from build123d import *

# Parameters (mm, degrees)
F0_W     = 82.55
F0_H     = 69.85
F1_DEPTH = 2.032
F2_W     = 1.524
F2_H     = 69.85
F3_DEPTH = 1.016
F5_DEPTH = 88.8746


with BuildPart() as f1:
    # F0 (on Top) → F1 (new body)
    with BuildSketch(Plane.XY):
        with Locations((-16.0199867169, 0.6959252059)):
            Rectangle(F0_W, F0_H)
    extrude(amount=F1_DEPTH)

    # F2 (on face) → F3 (join)
    with BuildSketch(Plane.XY.offset(2.032)):
        with Locations((-56.5329867169, 0.6959252059)):
            Rectangle(F2_W, F2_H)
        with Locations((-47.5413867169, 0.6959252059)):
            Rectangle(F2_W, F2_H)
        with Locations((-38.5497867169, 0.6959252059)):
            Rectangle(F2_W, F2_H)
        with Locations((-29.5581867169, 0.6959252059)):
            Rectangle(F2_W, F2_H)
        with Locations((-20.5665867169, 0.6959252059)):
            Rectangle(F2_W, F2_H)
        with Locations((-11.5749867169, 0.6959252059)):
            Rectangle(F2_W, F2_H)
        with Locations((-2.5833867169, 0.6959252059)):
            Rectangle(F2_W, F2_H)
        with Locations((6.4082132831, 0.6959252059)):
            Rectangle(F2_W, F2_H)
        with Locations((15.3998132831, 0.6959252059)):
            Rectangle(F2_W, F2_H)
        with Locations((24.3914132831, 0.6959252059)):
            Rectangle(F2_W, F2_H)
    extrude(amount=F3_DEPTH)

    # F4 (on face) → F5 (cut)
    with BuildSketch(Plane.YZ.offset(25.2550132831)):
        Polygon((33.9077030866, 0), (33.703327179, -0.3639321658), (35.670414567, -0.3639321658), (35.670414567, 3.138860222), (35.048827404, 2.032), (35.6209252059, 2.032), (35.6209252059, 0), align=None)
        Polygon((35.048827404, 2.032), (33.9077030866, 0), (35.6209252059, 0), (35.6209252059, 2.032), align=None)
    extrude(amount=-F5_DEPTH, mode=Mode.SUBTRACT)


solid = f1.part
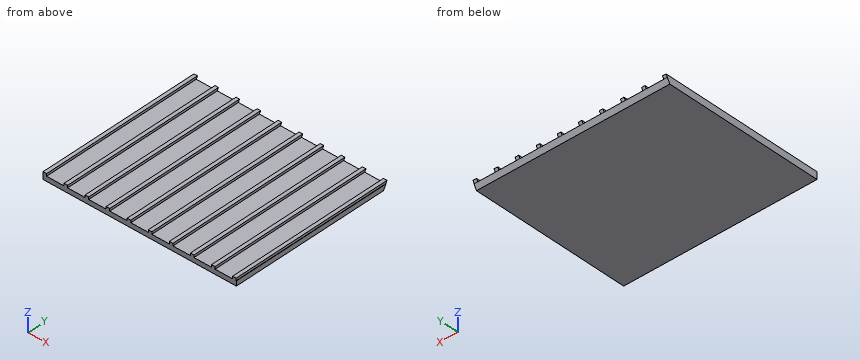
Geometry check sheet. Reference: the model listing, model coordinates, mm. Coordinates: 2 decimals unless noted, no trailing zeros. Order: outer loops, then holes, each group sorted by start corner. A loop starts at its lowest first (then second) coordinate and runs counter-clockwise, first axis right, second up. Notation, with made-up numbers: (29, 69.5) -> (66, 69.5) arc R16 ccw to (66, 77.5) -> close; hole circle Ø6 at (-11.75, 76). An arc over 180 degrees is marked (long way). Use a Markdown table: item, result. Add a question column.
1. Go/stop test with flat-tipped pins: pin 1 Ø1 at (x, z) = (-26, 0.5) entering from +Y; pin 2 Ø4 at (x, y) = (-31.5, 26.5) entering from +Z; pin 3 Ø2 at (x, y) = (21.5, 13.5) entering from +Z; pin 4 Ø0.5 at (y, z) = (-8.5, 2.5) entering from +X. Record where each tip stops, or that it passes through.
2. Cross-section at A-A (x = -49.5). Enter the section's corners in (y, z).
3. Cross-section at B-B (z = 0.8). Enter the section's corners in (x, y), and give its area (3 significant figures).
4. Material ranges on L1, parallel to Z at x = -27, y = 23; L2, parallel to Y at x = 10, z = 0.8; L3, parallel to Y at x = 5, z = 0.5, recorded low to high.
Filled sheet:
| question | item | result |
|---|---|---|
| 1 | pin 1 | y = 34.47 |
| 1 | pin 2 | z = 3.05 |
| 1 | pin 3 | z = 2.03 |
| 1 | pin 4 | x = 25.15 |
| 2 | outline | (-34.23, 0) -> (33.91, 0) -> (35.05, 2.03) -> (-34.23, 2.03) -> close |
| 3 | outline | (-57.29, -34.23) -> (25.26, -34.23) -> (25.26, 34.36) -> (-57.29, 34.36) -> close |
| 3 | area | 5,660 mm2 |
| 4 | L1 | 0 to 2.03 |
| 4 | L2 | -34.23 to 34.36 |
| 4 | L3 | -34.23 to 34.19 |
